Here's how the part is built. I have some questions about the finished solid (model axes, mm). A direction names the side the tool comes from. Round coordinates to 2 decimals unless told otherwise and drop trailing zeros. Write each loop counter-clockwise with the first axis right and the second up, starting at its lowest first coordinate (ties: lowest second). Pieces come first, ordered by that corner, then holes. Notation, with made-up numbers: (30, -33.5) -> (84, -33.5) arc R17 ccw to (84, -29.5) -> close; hole circle Ø4 at (16.25, 14). An arc over 180 degrees is marked (long way). Answer in a Markdown table with one row per item.
from build123d import *

# Parameters (mm, degrees)
SKETCH1_W          = 100
SKETCH1_H          = 50
BASE_FLANGE1_DEPTH = 2
SKETCH8_R          = 3.25
CUT_EXTRUDE1_DEPTH = 56.937465084
EDGE_FLANGE1_DEPTH = 50
EDGE_FLANGE2_DEPTH = 50
CUT_EXTRUDE2_DEPTH = 104.736569821
CUT_EXTRUDE3_DEPTH = 104.736569821
LPATTERN1_COUNT    = 3
LPATTERN1_PITCH    = 20
FILLET1_R          = 5


# Sheet-metal steps are written as plain solids
with BuildPart() as part:
    # Sketch1 → Base-Flange1 (new body)
    with BuildSketch(Plane(origin=(0, 0, 0), x_dir=(1, 0, 0), z_dir=(0, 1, 0))):
        Rectangle(SKETCH1_W, SKETCH1_H)
    extrude(amount=-BASE_FLANGE1_DEPTH)

    # Sketch8 → Cut-Extrude1 (cut, through all)
    with BuildSketch(Plane(origin=(0, 0, 0), x_dir=(1, 0, 0), z_dir=(0, 1, 0))):
        with Locations(Location((0, 0, 0), (0, 0, 270))):
            Circle(SKETCH8_R)
    extrude(amount=-CUT_EXTRUDE1_DEPTH, mode=Mode.SUBTRACT)

    # Edge-Flange1 section (across the edge) → Edge-Flange1 (add)
    with BuildSketch(Plane(origin=(50, -2, 25.7366), x_dir=(0, 0, -1), z_dir=(-1, 0, 0))):
        with BuildLine():
            Line((-2, 0.7366), (-2, 70))
            Line((-2, 70), (0, 70))
            Line((0, 70), (0, 0.7366))
            ThreePointArc((0, 0.7366), (0.215745145, 0.215745145), (0.7366, 0))
            Line((0.7366, 0), (0.7366, -2))
            ThreePointArc((0.7366, -2), (-1.198468417, -1.198468417), (-2, 0.7366))
        make_face()
    extrude(amount=EDGE_FLANGE1_DEPTH)

    # Edge-Flange2 section (across the edge) → Edge-Flange2 (add)
    with BuildSketch(Plane(origin=(-50, -2, -25.7366), x_dir=(0, 0, 1), z_dir=(1, 0, 0))):
        with BuildLine():
            Line((-2, 0.7366), (-2, 38))
            Line((-2, 38), (0, 38))
            Line((0, 38), (0, 0.7366))
            ThreePointArc((0, 0.7366), (0.215745145, 0.215745145), (0.7366, 0))
            Line((0.7366, 0), (0.7366, -2))
            ThreePointArc((0.7366, -2), (-1.198468417, -1.198468417), (-2, 0.7366))
        make_face()
    extrude(amount=EDGE_FLANGE2_DEPTH)

    # Sketch12 → Cut-Extrude2 (cut, through all)
    with BuildSketch(Plane.XY.offset(27.7366)):
        with BuildLine():
            Line((28.3, -55), (28.3, -59))
            ThreePointArc((28.3, -59), (25, -62.3), (21.7, -59))
            Line((21.7, -59), (21.7, -55))
            ThreePointArc((21.7, -55), (25, -51.7), (28.3, -55))
        make_face()
    cut_extrude2 = extrude(amount=-CUT_EXTRUDE2_DEPTH, mode=Mode.SUBTRACT)

    # Sketch16 → Cut-Extrude3 (cut, through all)
    with BuildSketch(Plane(origin=(0, 0, -27.7366), x_dir=(-1, 0, 0), z_dir=(0, 0, -1))):
        with BuildLine():
            Line((21.5, -25), (21.5, -15))
            ThreePointArc((21.5, -15), (25, -11.5), (28.5, -15))
            Line((28.5, -15), (28.5, -25))
            ThreePointArc((28.5, -25), (25, -28.5), (21.5, -25))
        make_face()
    extrude(amount=-CUT_EXTRUDE3_DEPTH, mode=Mode.SUBTRACT)

    # LPattern1: Cut-Extrude2 ×3
    with Locations(*[(0, i * LPATTERN1_PITCH, 0) for i in range(1, LPATTERN1_COUNT)]):
        add(cut_extrude2, mode=Mode.SUBTRACT)

    # Fillet1
    fillet1_edges = [part.edges().sort_by_distance(p)[0] for p in [
        (50, -72, 26.7366),
        (0, -72, 26.7366),
        (-50, -1, 25),
        (50, -1, -25),
        (-50, -40, -26.7366),
        (0, -40, -26.7366),
    ]]
    fillet(fillet1_edges, radius=FILLET1_R)


solid = part.part
1) We'd pull the mould along X, two halves only. Please class faces 1 (the face through (-31, -22, -25.737)), 2 (the face through (25.1, -22.3, 26.8)), 3 (the face through (49, -70, 27)): +X half, -X half, draft (parallel to the pull), parting line (faces both ways), or undercut.
Response:
| item | result |
|---|---|
| face 1 | draft |
| face 2 | undercut |
| face 3 | +X half |
2) I want a section at A-A, the plane x = -25. List the corners of the cut face in (y, z) for me.
Response:
| item | result |
|---|---|
| outline | (-40, -27.74) -> (-28.5, -27.74) -> (-28.5, -25.74) -> (-40, -25.74) -> close; (-11.5, -27.74) -> (-2.74, -27.74) arc R2.74 ccw to (0, -25) -> (0, 25) -> (-2, 25) -> (-2, -25) arc R0.74 cw to (-2.74, -25.74) -> (-11.5, -25.74) -> close |
3) I need wall thicknesses on line 1 (X direction, y = -0.8, z = 0); line 2 (Y direction, x = -16, z = 0.5); line 3 (Z direction, x = -37.5, y = -16). Which ranges of each line are inside material? Lowest first, please. Write a range as [from, to].
Response:
| item | result |
|---|---|
| line 1 | x = [-50, -3.25], [3.25, 50] |
| line 2 | y = [-2, 0] |
| line 3 | z = [-27.74, -25.74] |
4) Which directions (+Z, -Z, +X, -X, +Y, -Y) give clear straight access to the entire face, cutting with the end or side of a thin tool? Please do faces 4 (the face through (0, -34, 27)), 5 (the face through (-25.1, -28.5, -26.8)), 6 (the face through (-1, -2, -6)), 7 (the face through (-50, -1, -14)).
Response:
| item | result |
|---|---|
| face 4 | +Z, -X, +Y, -Y |
| face 5 | +Z, -Z |
| face 6 | +X, -X, -Y |
| face 7 | +Z, -Z, -X, +Y, -Y |
5) I want a section at B-B, the plane z = 0. List the corners of the cut face in (x, y) for me.
Response:
| item | result |
|---|---|
| outline | (-50, -2) -> (-3.25, -2) -> (-3.25, 0) -> (-50, 0) -> close; (3.25, -2) -> (50, -2) -> (50, 0) -> (3.25, 0) -> close |
6) I want a section at D-D, the plane z = 11. List the corners of the cut face in (x, y) for me.
Response:
| item | result |
|---|---|
| outline | (-50, -2) -> (50, -2) -> (50, 0) -> (-50, 0) -> close |
7) For pin 1 (1.6 mm diameter, centred on y = -17.5, z = 27, fed in from -X); pin 2 (15 mm diameter, centred on x = 9, z = -11, fed in from -Y); pin 3 (15 mm diameter, centred on x = 13, y = -45, fed in from -Z), each with a flat end and sliding along its axis, tell me the tip position at first contact or that it passes through.
Response:
| item | result |
|---|---|
| pin 1 | stops at x = 0 |
| pin 2 | stops at y = -2 |
| pin 3 | stops at z = 25.74 |
8) I want a section at C-C, the plane x = 25. List the corners of the cut face in (y, z) for me.
Response:
| item | result |
|---|---|
| outline | (-72, 25.74) -> (-62.3, 25.74) -> (-62.3, 27.74) -> (-72, 27.74) -> close; (-51.7, 25.74) -> (-42.3, 25.74) -> (-42.3, 27.74) -> (-51.7, 27.74) -> close; (-31.7, 25.74) -> (-22.3, 25.74) -> (-22.3, 27.74) -> (-31.7, 27.74) -> close; (-11.7, 25.74) -> (-2.74, 25.74) arc R0.74 cw to (-2, 25) -> (-2, -25) -> (0, -25) -> (0, 25) arc R2.74 ccw to (-2.74, 27.74) -> (-11.7, 27.74) -> close |
